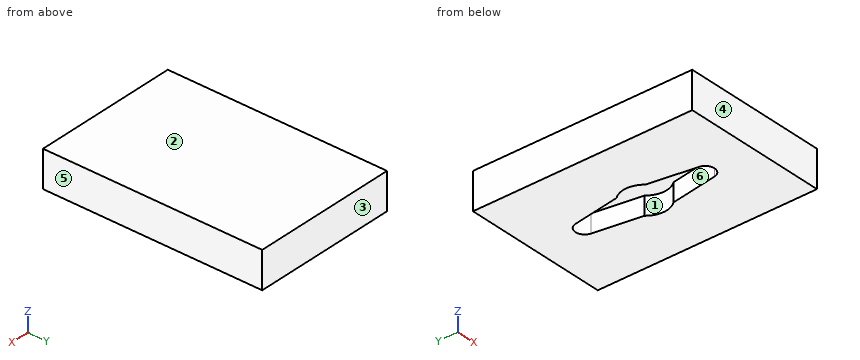
from build123d import *

# Parameters (mm, degrees)
ESQUISSE2_W        = 40
ESQUISSE2_H        = 60
BOSS_EXTRU_1_DEPTH = 5
ESQUISSE3_W        = 40
ESQUISSE3_H        = 60
BOSS_EXTRU_2_DEPTH = 5


with BuildPart() as part:
    # Esquisse2 → Boss.-Extru.1 (new body)
    with BuildSketch(Plane.XY):
        with Locations((5, -165.745255904)):
            Rectangle(ESQUISSE2_W, ESQUISSE2_H)
        with BuildLine():
            Line((9.5, -169.713882871), (7.469689731, -182.633370102))
            ThreePointArc((7.469689731, -182.633370102), (5, -184.745255904), (2.530310269, -182.633370102))
            Line((2.530310269, -182.633370102), (0.5, -169.713882871))
            ThreePointArc((0.5, -169.713882871), (-1, -165.745255904), (0.5, -161.776628937))
            Line((0.5, -161.776628937), (2.530310269, -148.857141706))
            ThreePointArc((2.530310269, -148.857141706), (5, -146.745255904), (7.469689731, -148.857141706))
            Line((7.469689731, -148.857141706), (9.5, -161.776628937))
            ThreePointArc((9.5, -161.776628937), (11, -165.745255904), (9.5, -169.713882871))
        make_face(mode=Mode.SUBTRACT)
    extrude(amount=BOSS_EXTRU_1_DEPTH)

    # Esquisse3 → Boss.-Extru.2 (add)
    with BuildSketch(Plane.XY.offset(5)):
        with Locations((5, -165.745255904)):
            Rectangle(ESQUISSE3_W, ESQUISSE3_H)
    extrude(amount=BOSS_EXTRU_2_DEPTH)


solid = part.part
Geometry: final body of the model. Coordinates: model frame, mm. Face numbers are marked on the shaded views. A direction names the side the tool comes from. Give positions to 0.01 mm unless a question says otherwise; leave off trailing zeros. Write each loop counter-clockwise with the first axis right and the second up, starting at its lowest first coordinate (ties: lowest second). Pieces come first, ordered by that corner, then holes. Notation, with made-up numbers: (-9, -27) - (10, -27) arc R9 cw to (10, -21) - close; hole circle Ø5 at (83.5, -5.75). An arc over 180 degrees is marked (long way). Return JSON: item names as keys, results as strings. Group by question number.
1) Section C-C on y = -175. Return the cut outline in (x, z).
2) Line query: line 1 (Y direction, x = 5, z = 2.5); line 2 (X direction, y = -148, z = 1.75); line 3 (X direction, y = -182.5, z = 3.5). Output: solid intervals per line, ascending.
3) Mould query, pull axis Y, two halves, no side actions, for the marked faces 1, 2, 3 and 4. Classes: released by +Y, released by -Y, zero draft, split by the parting line, or undercut.
4) Section A-A on z = 3. Return the cut outline in (x, y), plus the area to 3 significant figures.
5) Set-up query: the marked faces 5 and 6. Return all of +Z, -Z, +X, -X, +Y, -Y with unobstructed straight access to the full face (end or side cutting, diameter ignored); none if empty.
6) Section B-B on y = -158. Return the cut outline in (x, z), plus the area to 3 significant figures.
Filled in:
{
 "1": {"outline": "(-15, 0) - (1.33, 0) - (1.33, 5) - (8.67, 5) - (8.67, 0) - (25, 0) - (25, 10) - (-15, 10) - close"},
 "2": {"line 1": "y = -195.75 to -184.75, -146.75 to -135.75", "line 2": "x = -15 to 2.83, 7.17 to 25", "line 3": "x = -15 to 2.51, 7.49 to 25"},
 "3": {"face 1": "undercut", "face 2": "zero draft", "face 3": "released by +Y", "face 4": "released by -Y"},
 "4": {"outline": "(-15, -195.75) - (25, -195.75) - (25, -135.75) - (-15, -135.75) - close; hole (0.5, -169.71) - (2.53, -182.63) arc R2.5 ccw to (7.47, -182.63) - (9.5, -169.71) arc R6 ccw to (9.5, -161.78) - (7.47, -148.86) arc R2.5 ccw to (2.53, -148.86) - (0.5, -161.78) arc R6 ccw to start", "area": "2,120 mm^2"},
 "5": {"face 5": "+Z, -Z, +X, +Y, -Y", "face 6": "-Z"},
 "6": {"outline": "(-15, 0) - (1.09, 0) - (1.09, 5) - (8.91, 5) - (8.91, 0) - (25, 0) - (25, 10) - (-15, 10) - close", "area": "361 mm^2"}
}
